Read the model definition and answer for the solid it produces. Units are mm, in the model's axes. Face numbers are marked on the shaded views. A direction names the side the tool comes from. Round coordinates to 2 decimals unless told otherwise and drop trailing zeros. Write each loop counter-clockwise with the first axis right and the second up, starting at its lowest first coordinate (ties: lowest second). Pieces come first, ordered by that corner, then holes. Notation, with made-up numbers: M 31,6.25 L 75,6.25 A15 ccw 75,32.25 Z; hole C 78,1 d2. An arc over 180 degrees is marked long. Use one line per item in the form item = value. Start each with the question number.
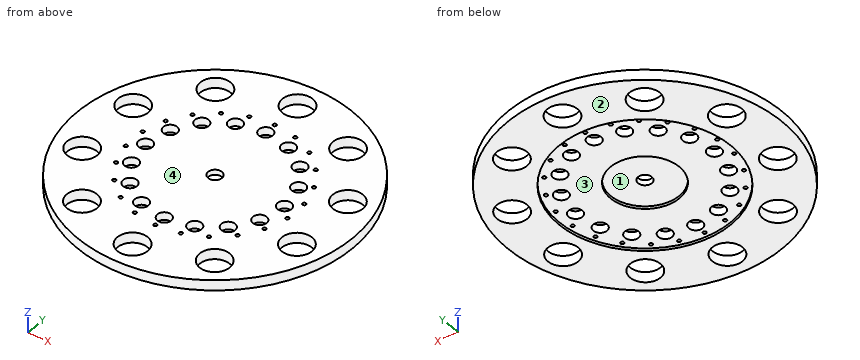
```python
from build123d import *

# Parameters (mm, degrees)
SKETCH1_R           = 80
BOSS_EXTRUDE1_DEPTH = 6
SKETCH2_R           = 20
CUT_EXTRUDE1_DEPTH  = 3
SKETCH3_R           = 8.810326898
CUT_EXTRUDE3_DEPTH  = 6
SKETCH5_R           = 50
CUT_EXTRUDE5_DEPTH  = 1.5
SKETCH6_R           = 1
SKETCH6_R_2         = 4
CUT_EXTRUDE6_DEPTH  = 6
SKETCH7_R           = 4
CUT_EXTRUDE8_DEPTH  = 6


with BuildPart() as part:
    # Sketch1 → Boss-Extrude1 (new body)
    with BuildSketch(Plane.XY):
        Circle(SKETCH1_R)
    extrude(amount=BOSS_EXTRUDE1_DEPTH)

    # Sketch2 → Cut-Extrude1 (cut)
    with BuildSketch(Plane(origin=(0, 0, 0), x_dir=(-1, 0, 0), z_dir=(0, 0, -1))):
        Circle(SKETCH2_R)
    extrude(amount=-CUT_EXTRUDE1_DEPTH, mode=Mode.SUBTRACT)

    # Sketch3 → Cut-Extrude3 (cut)
    with BuildSketch(Plane(origin=(0, 0, 0), x_dir=(-1, 0, 0), z_dir=(0, 0, -1))):
        with Locations((0, 65)):
            Circle(SKETCH3_R)
        with Locations((38.206041399, 52.586104634)):
            Circle(SKETCH3_R)
        with Locations((61.818673559, 20.086104634)):
            Circle(SKETCH3_R)
        with Locations((61.818673559, -20.086104634)):
            Circle(SKETCH3_R)
        with Locations((38.206041399, -52.586104634)):
            Circle(SKETCH3_R)
        with Locations((0, -65)):
            Circle(SKETCH3_R)
        with Locations((-38.206041399, -52.586104634)):
            Circle(SKETCH3_R)
        with Locations((-61.818673559, -20.086104634)):
            Circle(SKETCH3_R)
        with Locations((-61.818673559, 20.086104634)):
            Circle(SKETCH3_R)
        with Locations((-38.206041399, 52.586104634)):
            Circle(SKETCH3_R)
    extrude(amount=-CUT_EXTRUDE3_DEPTH, mode=Mode.SUBTRACT)

    # Sketch5 → Cut-Extrude5 (cut)
    with BuildSketch(Plane(origin=(0, 0, 0), x_dir=(-1, 0, 0), z_dir=(0, 0, -1))):
        Circle(SKETCH5_R)
    extrude(amount=-CUT_EXTRUDE5_DEPTH, mode=Mode.SUBTRACT)

    # Sketch6 → Cut-Extrude6 (cut)
    with BuildSketch(Plane(origin=(0, 0, 1.5), x_dir=(-1, 0, 0), z_dir=(0, 0, -1))):
        with Locations((0, 47)):
            Circle(SKETCH6_R)
        with Locations((13.241430172, 45.09616976)):
            Circle(SKETCH6_R)
        with Locations((25.41011842, 39.538916043)):
            Circle(SKETCH6_R)
        with Locations((35.520229995, 30.778454495)):
            Circle(SKETCH6_R)
        with Locations((42.752703782, 19.524505611)):
            Circle(SKETCH6_R)
        with Locations((46.521607768, 6.688797399)):
            Circle(SKETCH6_R)
        with Locations((46.521607768, -6.688797399)):
            Circle(SKETCH6_R)
        with Locations((42.752703782, -19.524505611)):
            Circle(SKETCH6_R)
        with Locations((35.520229995, -30.778454495)):
            Circle(SKETCH6_R)
        with Locations((25.41011842, -39.538916043)):
            Circle(SKETCH6_R)
        with Locations((13.241430172, -45.09616976)):
            Circle(SKETCH6_R)
        with Locations((0, -47)):
            Circle(SKETCH6_R)
        with Locations((-13.241430172, -45.09616976)):
            Circle(SKETCH6_R)
        with Locations((-25.41011842, -39.538916043)):
            Circle(SKETCH6_R)
        with Locations((-35.520229995, -30.778454495)):
            Circle(SKETCH6_R)
        with Locations((-42.752703782, -19.524505611)):
            Circle(SKETCH6_R)
        with Locations((-46.521607768, -6.688797399)):
            Circle(SKETCH6_R)
        with Locations((-46.521607768, 6.688797399)):
            Circle(SKETCH6_R)
        with Locations((-42.752703782, 19.524505611)):
            Circle(SKETCH6_R)
        with Locations((-35.520229995, 30.778454495)):
            Circle(SKETCH6_R)
        with Locations((-25.41011842, 39.538916043)):
            Circle(SKETCH6_R)
        with Locations((-13.241430172, 45.09616976)):
            Circle(SKETCH6_R)
        with Locations((0, 40)):
            Circle(SKETCH6_R_2)
        with Locations((15.307337295, 36.9551813)):
            Circle(SKETCH6_R_2)
        with Locations((28.284271247, 28.284271247)):
            Circle(SKETCH6_R_2)
        with Locations((36.9551813, 15.307337295)):
            Circle(SKETCH6_R_2)
        with Locations((40, 0)):
            Circle(SKETCH6_R_2)
        with Locations((36.9551813, -15.307337295)):
            Circle(SKETCH6_R_2)
        with Locations((28.284271247, -28.284271247)):
            Circle(SKETCH6_R_2)
        with Locations((15.307337295, -36.9551813)):
            Circle(SKETCH6_R_2)
        with Locations((0, -40)):
            Circle(SKETCH6_R_2)
        with Locations((-15.307337295, -36.9551813)):
            Circle(SKETCH6_R_2)
        with Locations((-28.284271247, -28.284271247)):
            Circle(SKETCH6_R_2)
        with Locations((-36.9551813, -15.307337295)):
            Circle(SKETCH6_R_2)
        with Locations((-40, 0)):
            Circle(SKETCH6_R_2)
        with Locations((-36.9551813, 15.307337295)):
            Circle(SKETCH6_R_2)
        with Locations((-28.284271247, 28.284271247)):
            Circle(SKETCH6_R_2)
        with Locations((-15.307337295, 36.9551813)):
            Circle(SKETCH6_R_2)
    extrude(amount=-CUT_EXTRUDE6_DEPTH, mode=Mode.SUBTRACT)

    # Sketch7 → Cut-Extrude8 (cut)
    with BuildSketch(Plane(origin=(0, 0, 3), x_dir=(-1, 0, 0), z_dir=(0, 0, -1))):
        Circle(SKETCH7_R)
    extrude(amount=-CUT_EXTRUDE8_DEPTH, mode=Mode.SUBTRACT)


solid = part.part
```
Q1. Straight lines are drawn through the part: line 1 (Y direction, x = -60, z = 3.8); line 2 (X direction, y = 25, z = 1.95); line 3 (X direction, y = 16, z = 2.4). For each, find the intervals that lie inside material, in ascending order. Write a range as [from, to].
Q2. Each of these flat-tipped pins is pushed along its axis until it touches: pin 1 Ø1.6 at (x, y) = (13.24, 45.1) entering from +Z; pin 2 Ø3 at (x, z) = (8.5, 1) entering from +Y; pin 3 Ø3 at (y, z) = (-35.5, 2.5) entering from -X; pin 4 Ø6 at (x, y) = (-4, -23.5) entering from -Z. Where does it stop, or does it pass through?
Q3. Find section C-C on y = -65. Write down the section's boundary in (x, z), and give its area (3 significant figures).
Q4. For a pull along X with two mould halves and no side action, classify the marked faces 3 and 4 as +X half, -X half, draft (parallel to the pull), parting line (faces both ways), or undercut.
Q5. Find section A-A on y = 0. Write down the section's boundary in (x, z).
Q6. Find section D-D on y = 68.5. Write down the section's boundary in (x, z).
Q7. A tool of negligible diameter and unlimited length cuts with its end or side. For the marked faces 1 and 2, from which of +Z, -Z, +X, -X, +Y, -Y can it reach the whole face along a straight path? Write none if from no direction.
Q8. Find section B-B on x = -62. Write down the section's boundary in (y, z).
Response:
q1.line_1 = [-52.92, -28.71], [-11.47, 11.47], [28.71, 52.92]
q1.line_2 = [-75.99, -69.13], [-54.51, -30.57], [-26, 26], [30.57, 54.51], [69.13, 75.99]
q1.line_3 = [-78.38, -69.62], [-54.01, -40.89], [-33.02, -12], [12, 33.02], [40.89, 54.01], [69.62, 78.38]
q2.pin_1 = through
q2.pin_2 = 79.69
q2.pin_3 = -72.42
q2.pin_4 = 1.5
q3.outline = M -46.64,0 L -8.81,0 L -8.81,6 L -46.64,6 Z; M 8.81,0 L 46.64,0 L 46.64,6 L 8.81,6 Z
q3.area = 454 mm²
q4.face_3 = undercut
q4.face_4 = draft
q5.outline = M -80,0 L -50,0 L -50,1.5 L -44,1.5 L -44,6 L -80,6 Z; M -36,1.5 L -20,1.5 L -20,3 L -4,3 L -4,6 L -36,6 Z; M 4,3 L 20,3 L 20,1.5 L 36,1.5 L 36,6 L 4,6 Z; M 44,1.5 L 50,1.5 L 50,0 L 80,0 L 80,6 L 44,6 Z
q6.outline = M -41.32,0 L -8.09,0 L -8.09,6 L -41.32,6 Z; M 8.09,0 L 41.32,0 L 41.32,6 L 8.09,6 Z
q7.face_1 = -Z
q7.face_2 = -Z, +X, -X, +Y, -Y
q8.outline = M -50.56,0 L -28.89,0 L -28.89,6 L -50.56,6 Z; M -11.28,0 L 11.28,0 L 11.28,6 L -11.28,6 Z; M 28.89,0 L 50.56,0 L 50.56,6 L 28.89,6 Z
